The model under review builds one solid part; all positions refer to its coordinate system, in mm. Give positions to 0.01 mm unless a question says otherwise; leave off trailing zeros. Order: outer loops, then holes, each group sorted by start corner. A loop starts at its lowest first (then second) coordinate and runs counter-clockwise, first axis right, second up. Notation, with made-up numbers: (21, 10) - (76, 10) arc R22 cw to (76, 37) - close; hole circle Ø5 at (6.5, -13.5). An arc over 180 degrees is marked (long way). Use CSV: the item, a comma, the result in double quotes. Start each with the question number.
1. Take a section at A-A, the plane z = 0. State the section outline as (x, y) points.
2. Take a section at B-B, the plane y = 2.3. State the section outline as (x, z) points.
3. Take a section at D-D, the plane x = 16. State the section outline as (y, z) points, then the cut area to 3 significant figures.
4. Take a section at C-C, the plane x = 7.5. State the section outline as (y, z) points, then the cut area to 3 significant figures.
5. Draft analysis for pull direction Z (two halves, no side actions). For faces 1 (the flat face through (0, 0, 0)), 2 (the cylindrical face through (-19.524, 2.465, -4.336)), 3 (the cylindrical face through (9.397, 1.521, 1.21)), state which applies: released by +Z, released by -Z, zero draft, split by the parting line, or undercut.
6. To check wall thickness, follow line 1 (X direction, y = 1.85, z = 0); line 2 (X direction, y = 3.4, z = 2); line 3 (X direction, y = 1.05, z = -7.5). State the ranges of each line that lie inside material, in increasing order. Write a range as [from, to].
7. For pin 1 (2 mm diameter, centred on y = 1.5, z = 5.5, fed in from -X); pin 2 (3 mm diameter, centred on x = 3, y = 0.5, fed in from +Z), all flat-tipped, find the tip position at first contact; note any pin that passes through.
```python
from build123d import *

# Parameters (mm, degrees)
SKETCH1_R           = 20
BOSS_EXTRUDE1_DEPTH = 5
SKETCH2_R           = 2.25
CUT_EXTRUDE1_DEPTH  = 5
CHAMFER1_SIZE       = 2


with BuildPart() as part:
    # Sketch1 → Boss-Extrude1 (new body)
    with BuildSketch(Plane(origin=(0, 0, 0), x_dir=(1, 0, 0), z_dir=(0, 1, 0))):
        with Locations(Location((0, 0, 0), (0, 0, 270))):
            Circle(SKETCH1_R)
    extrude(amount=BOSS_EXTRUDE1_DEPTH)

    # Sketch2 → Cut-Extrude1 (cut)
    with BuildSketch(Plane(origin=(0, 5, 0), x_dir=(1, 0, 0), z_dir=(0, 1, 0))):
        with Locations(Location((-7.5, 0, 0), (0, 0, 270))):
            Circle(SKETCH2_R)
        with Locations(Location((7.5, 0, 0), (0, 0, 270))):
            Circle(SKETCH2_R)
    extrude(amount=-CUT_EXTRUDE1_DEPTH, mode=Mode.SUBTRACT)

    # Chamfer1
    chamfer1_edges = [part.edges().sort_by_distance(p)[0] for p in [
        (7.5, 5, -2.25),
        (-7.5, 5, -2.25),
    ]]
    chamfer(chamfer1_edges, length=CHAMFER1_SIZE)


solid = part.part
```
Determined:
1,outline,"(-20, 0) - (-9.75, 0) - (-9.75, 3) - (-11.75, 5) - (-20, 5) - close; (-5.25, 0) - (5.25, 0) - (5.25, 3) - (3.25, 5) - (-3.25, 5) - (-5.25, 3) - close; (9.75, 0) - (20, 0) - (20, 5) - (11.75, 5) - (9.75, 3) - close"
2,outline,"circle Ø40 at (0, 0); hole circle Ø4.5 at (-7.5, 0); hole circle Ø4.5 at (7.5, 0)"
3,outline,"(0, -12) - (5, -12) - (5, 12) - (0, 12) - close"
3,area,"120 mm²"
4,outline,"(0, -18.54) - (5, -18.54) - (5, -4.25) - (3, -2.25) - (0, -2.25) - close; (0, 2.25) - (3, 2.25) - (5, 4.25) - (5, 18.54) - (0, 18.54) - close"
4,area,"159 mm²"
5,face 1,"zero draft"
5,face 2,"split by the parting line"
5,face 3,"undercut"
6,line 1,"x = [-20, -9.75], [-5.25, 5.25], [9.75, 20]"
6,line 2,"x = [-19.9, -9.24], [-5.76, 5.76], [9.24, 19.9]"
6,line 3,"x = [-18.54, 18.54]"
7,pin 1,"stops at x = -19.49"
7,pin 2,"stops at z = 19.94"
